from build123d import *

# Parameters (mm, degrees)
EXTRUDE_3_DEPTH     = 20
CUT_EXTRUDE_4_DEPTH = 15
CUT_EXTRUDE_START   = -5
SKETCH_6_R          = 2.52
CUT_EXTRUDE_5_DEPTH = 5


with BuildPart() as part:
    # 草图1 → 凸台-拉伸3 (new body)
    with BuildSketch(Plane(origin=(0, 0, 0), x_dir=(1, 0, 0), z_dir=(0, 1, 0))):
        with BuildLine():
            Line((9.98, -2.98), (5.184592559, -2.98))
            ThreePointArc((5.184592559, -2.98), (0, -5.98), (-5.184592559, -2.98))
            Line((-5.184592559, -2.98), (-9.98, -2.98))
            Line((-9.98, -2.98), (-9.98, 2.98))
            Line((-9.98, 2.98), (-5.184592559, 2.98))
            ThreePointArc((-5.184592559, 2.98), (0, 5.98), (5.184592559, 2.98))
            Line((5.184592559, 2.98), (9.98, 2.98))
            Line((9.98, 2.98), (9.98, -2.98))
        make_face()
    extrude(amount=EXTRUDE_3_DEPTH)

    # 草图5 → 切除-拉伸4 (cut)
    with BuildSketch(Plane(origin=(0, 20, 0), x_dir=(1, 0, 0), z_dir=(0, 1, 0))):
        with BuildLine():
            Line((-2.009975124, 1.52), (2.009975124, 1.52))
            ThreePointArc((2.009975124, 1.52), (0, -2.52), (-2.009975124, 1.52))
        make_face()
    extrude(amount=-CUT_EXTRUDE_4_DEPTH, mode=Mode.SUBTRACT)

    # 草图6 → 切除-拉伸5 (cut)
    with BuildSketch(Plane.XZ.offset(CUT_EXTRUDE_START)):
        with Locations(Location((0, 0, 0), (0, 0, 217.097601801))):
            Circle(SKETCH_6_R)
    extrude(amount=CUT_EXTRUDE_5_DEPTH, mode=Mode.SUBTRACT)


solid = part.part
Check sheet for the modelled part. Datum: model origin and axes. Units: mm. A direction names the side the tool comes from. Round coordinates to 2 decimals unless told otherwise and drop trailing zeros. Loops run counter-clockwise (first coordinate to the right, second up) from the corner with the lowest first, then second, coordinate; pieces in that order, holes last. Notation, with made-up numbers: M -27.5,47.25 L -16.5,47.25 A13 ccw -16.5,53.25 Z; hole C 26.25,53 d3. An arc over 180 degrees is marked long. One line per question, with ' | ' between items. Start each with the question number.
Item 1: Section check B-B (z = 0). Record the boundary of the cut face in (x, y), and give its area (3 significant figures).
Item 2: Release check for a two-part mould opening along Z. For faces 1 (the face through (-9.98, 10, 0)), 2 (the face through (8, 10, -2.98)), 3 (the face through (0, 13, -1.52)) record: released by +Z, released by -Z, zero draft, split by the parting line, or undercut.
Item 3: Section check A-A (x = 0). Record the boundary of the cut face in (y, z).
Item 4: Section check D-D (x = 8.25). Record the boundary of the cut face in (y, z).
Item 5: Scan lines: probe 1 along X at (y, z) = (3.8, 0); probe 2 along Z at (x, y) = (6.75, 13.25); probe 3 along X at (y, z) = (11.25, -0.75). Record each from-to range of solid material in increasing order.
Item 6: Gauge pin test, flat ends, axial feed: pin 1 Ø0.5 at (x, z) = (0.5, -2) entering from -Y; pin 2 Ø1.4 at (x, y) = (-8, 7) entering from +Z; pin 3 Ø1.5 at (x, y) = (4.5, 11) entering from +Z. Record the tip position at first contact, or that the pin passes through.
Item 7: Section check C-C (y = 11.5). Record the boundary of the cut face in (x, z).
Item 8: Set-up check for faces 4 (the face through (8, 10, 2.98)), 5 (the face through (0, 5, -2)), 6 (the face through (-8, 10, -2.98)), 7 (the face through (0.09, 9.86, 5.98)), 8 (the face through (-8, 10, 2.98)): record each of +Z, -Z, +X, -X, +Y, -Y from which the full face is reachable in a straight line by a thin tool's end or side.
Worked out:
1) outline: M -9.98,0 L -2.52,0 L -2.52,20 L -9.98,20 Z; M 2.52,0 L 9.98,0 L 9.98,20 L 2.52,20 Z | area: 298 mm^2
2) face 1: zero draft | face 2: released by -Z | face 3: undercut
3) outline: M 0,-5.98 L 20,-5.98 L 20,-1.52 L 5,-1.52 L 5,-2.52 L 0,-2.52 Z; M 0,2.52 L 20,2.52 L 20,5.98 L 0,5.98 Z
4) outline: M 0,-2.98 L 20,-2.98 L 20,2.98 L 0,2.98 Z
5) probe 1: -9.98 to -2.52, 2.52 to 9.98 | probe 2: -2.98 to 2.98 | probe 3: -9.98 to -2.41, 2.41 to 9.98
6) pin 1: y = 5 | pin 2: z = 2.98 | pin 3: z = 4.66
7) outline: M -9.98,-2.98 L -5.18,-2.98 A5.98 ccw 5.18,-2.98 L 9.98,-2.98 L 9.98,2.98 L 5.18,2.98 A5.98 ccw -5.18,2.98 L -9.98,2.98 Z; hole M -2.01,-1.52 L 2.01,-1.52 A2.52 ccw long Z
8) face 4: +Z, +X, +Y, -Y | face 5: -Y | face 6: -Z, -X, +Y, -Y | face 7: +Z, +Y, -Y | face 8: +Z, -X, +Y, -Y
